Solid Edge part; units mm, degrees
sketch "Sketch1" plane through (0, 0, 0) normal (0, 0, 1) x (1, 0, 0)
  line L0 (-75, -25) -> (75, -25)
  line L1 (75, -25) -> (75, 25)
  line L2 (75, 25) -> (-75, 25)
  line L3 (-75, 25) -> (-75, -25)
extrude "Protrusion1" add sketch "Sketch1" against normal blind 60
sketch "Sketch2" plane through (0, -25, -30) normal (0, -1, 0) x (1, 0, 0)
  circle A0 centre (0, 30) radius 41
extrude "ExtrudedCutout_1" cut sketch "Sketch2" against normal blind 50
Here's how the part is built. I have some questions about the finished solid (model axes, mm). Give positions to 0.01 mm unless a question says otherwise; leave off trailing zeros. Order: outer loops, then holes, each group sorted by start corner. A loop starts at its lowest first (then second) coordinate and runs counter-clockwise, first axis right, second up. Notation, with made-up numbers: M -1.75,52 L 51.25,52 A33 ccw 51.25,88 Z; hole C 58,64.5 d6. An arc over 180 degrees is marked long. Answer as a JSON object with one key per item and string values. Group by question number.
1) I'm going to push a flat-ended pin straight in: pin 1 Ø3 at (x, y) = (20, 14.5) entering from +Z. Where does the tip first touch, or does it pass through?
2) Suppose I cut it at A-A, the plane z = -34. Write out the boundary of the cut face in (x, y).
3) Suppose I cut it at D-D, the plane x = 15.5. Write out the boundary of the cut face in (y, z), plus the area to 3 significant figures.
4) Suppose I cut it at B-B, the plane y = -10. Write out the boundary of the cut face in (x, z).
5) We'd pull the mould along X, two halves only. Please class faces 1 (the cylindrical face through (-0.9, -0.35, -40.99)), 2 (the flat face through (1, 25, -43)), 3 (the flat face through (75, 0, -30)): pulls with the +X half, pulls with the -X half, needs draft (parallel to the pull), parting line crosses it, or undercut.
6) Please list where these lines run through material, in increasing order: L1, parallel to X at y = -18.5, z = -14; L2, parallel to X at y = 2, z = -17; L3, parallel to Z at x = 34, y = 8.5. Write a range as [from, to].
7) Suppose I cut it at C-C, the plane x = 0. Write out the boundary of the cut face in (y, z).
Results found:
{
 "1": {"pin 1": "z = -34.91"},
 "2": {"outline": "M -75,-25 L -22.91,-25 L -22.91,25 L -75,25 Z; M 22.91,-25 L 75,-25 L 75,25 L 22.91,25 Z"},
 "3": {"outline": "M -25,-60 L 25,-60 L 25,-37.96 L -25,-37.96 Z", "area": "1,100 mm²"},
 "4": {"outline": "M -75,-60 L 75,-60 L 75,0 L 41,0 A41 cw -41,0 L -75,0 Z"},
 "5": {"face 1": "undercut", "face 2": "needs draft", "face 3": "pulls with the +X half"},
 "6": {"L1": "[-75, -38.54], [38.54, 75]", "L2": "[-75, -37.31], [37.31, 75]", "L3": "[-60, -22.91]"},
 "7": {"outline": "M -25,-60 L 25,-60 L 25,-41 L -25,-41 Z"}
}
